For this review, take the finished solid that the model builds, in its own axes (mm). A direction names the side the tool comes from. Coordinates: 2 decimals unless noted, no trailing zeros. Order: outer loops, then holes, each group sorted by start corner. A loop starts at its lowest first (then second) coordinate and runs counter-clockwise, first axis right, second up. Notation, with made-up numbers: (46.25, 58.5) -> (94.25, 58.5) arc R31 ccw to (94.25, 92.5) -> close; hole circle Ø4 at (42, 2). An arc over 180 degrees is marked (long way). Answer as a JSON object with one key per item and string values. Group by question number.
1) Machinability: for faces 4 (the flat face through (18.5, 0, -1)), 5 (the flat face through (-18.5, 0, -1)), 6 (the flat face through (-7.3, 17, 0)), which of the approach directions +Z, -Z, +X, -X, +Y, -Y give a long, thin tool a straight path to every point of the face, cutting with its end or side? Answer none if there is none.
2) Add section A-A, the plane y = 16. Write out the cut boundary in (x, z).
3) For pin 1 (0.6 mm diameter, centred on x = -8.5, z = -0.5, fed in from +Y); pin 2 (1.4 mm diameter, centred on y = -7, z = -1, fed in from -X), all flat-tipped, find the tip position at first contact; note any pin that passes through.
4) Add section B-B, the plane z = -0.85. Write out the cut boundary in (x, y).
5) Wall thickness on L1, parallel to X at y = 15, z = 0.6; L2, parallel to Y at x = 11.5, z = -1; L3, parallel to X at y = 0.5, z = -0.3: over which ranges is each line inside the solid? List them lowest first.
6) Add section C-C, the plane x = 2. Write out the cut boundary in (y, z), then the cut area to 3 significant figures.
7) Draft analysis for pull direction Y (two halves, no side actions). For faces 1 (the flat face through (0, -21, -1)), 2 (the flat face through (-8, 18.6, 0)), 3 (the flat face through (0, 0, -1.3)), state which applies: +Y half, -Y half, draft (parallel to the pull), parting line (faces both ways), or undercut.
from build123d import *

# Parameters (mm, degrees)
F1_DEPTH = 1.5
F2_W     = 37
F2_H     = 42
F3_DEPTH = 1.3
F4_W     = 2.1
F4_H     = 4
F5_DEPTH = 5.05


with BuildPart() as f1:
    # F0 (on Top) → F1 (new body)
    with BuildSketch(Plane.XY):
        with BuildLine():
            Line((17, 23.5), (-17, 23.5))
            ThreePointArc((-17, 23.5), (-19.12132, 22.62132), (-20, 20.5))
            Line((-20, 20.5), (-20, -20.5))
            ThreePointArc((-20, -20.5), (-19.12132, -22.62132), (-17, -23.5))
            Line((-17, -23.5), (17, -23.5))
            ThreePointArc((17, -23.5), (19.12132, -22.62132), (20, -20.5))
            Line((20, -20.5), (20, 20.5))
            ThreePointArc((20, 20.5), (19.12132, 22.62132), (17, 23.5))
        make_face()
    extrude(amount=F1_DEPTH)

    # F2 (on Top) → F3 (join)
    with BuildSketch(Plane.XY):
        Rectangle(F2_W, F2_H)
    extrude(amount=-F3_DEPTH)

    # F4 (on Top) → F5 (cut, symmetric)
    with BuildSketch(Plane.XY):
        with Locations((-8.35, 16.6)):
            Rectangle(F4_W, F4_H)
    extrude(amount=F5_DEPTH, both=True, mode=Mode.SUBTRACT)


solid = f1.part
Output values:
{
 "1": {"face 4": "-Z, +X, +Y, -Y", "face 5": "-Z, -X, +Y, -Y", "face 6": "+Z, -Z"},
 "2": {"outline": "(-20, 0) -> (-18.5, 0) -> (-18.5, -1.3) -> (-9.4, -1.3) -> (-9.4, 1.5) -> (-20, 1.5) -> close; (-7.3, -1.3) -> (18.5, -1.3) -> (18.5, 0) -> (20, 0) -> (20, 1.5) -> (-7.3, 1.5) -> close"},
 "3": {"pin 1": "stops at y = 21", "pin 2": "stops at x = -18.5"},
 "4": {"outline": "(-18.5, -21) -> (18.5, -21) -> (18.5, 21) -> (-18.5, 21) -> close; hole (-9.4, 14.6) -> (-7.3, 14.6) -> (-7.3, 18.6) -> (-9.4, 18.6) -> close"},
 "5": {"L1": "x = -20 to -9.4, -7.3 to 20", "L2": "y = -21 to 21", "L3": "x = -18.5 to 18.5"},
 "6": {"outline": "(-23.5, 0) -> (-21, 0) -> (-21, -1.3) -> (21, -1.3) -> (21, 0) -> (23.5, 0) -> (23.5, 1.5) -> (-23.5, 1.5) -> close", "area": "125 mm²"},
 "7": {"face 1": "-Y half", "face 2": "undercut", "face 3": "draft"}
}
